For this review, take the finished solid that the model builds, in its own axes (mm). A direction names the side the tool comes from. Coordinates: 2 decimals unless noted, no trailing zeros. Write each loop counter-clockwise with the first axis right and the second up, starting at its lowest first coordinate (ties: lowest second). Pieces come first, ordered by that corner, then holes. Notation, with made-up numbers: (19, 17) -> (32, 17) arc R35 ccw to (32, 55) -> close; hole circle Ø8 at (79.5, 87.25). An arc over 180 degrees is marked (long way). Put each result on its own line as item: value. Start each with the question number.
Item 1: To check wall thickness, follow L1, parallel to Y at x = -43.5, z = -18.5; L2, parallel to Z at x = -38.5, y = 4.25; L3, parallel to X at y = -1.25, z = -8. State the ranges of each line that lie inside material, in increasing order.
Item 2: For faces 4 (the flat face through (-21, 5, -17)), 5 (the flat face through (-37, 2, -24)), 6 (the flat face through (-40.7, 0, -14.2)), list the 3-axis set-ups (+Z, -Z, +X, -X, +Y, -Y) from which the entire face can be reached by the end or side of a thin tool; tool diameter is ignored.
Item 3: Consider section C-C on y = -6.75. Give the boundary of the cut face in (x, z).
Item 4: The part is to be moulded in two halves that separate along X. For faces 1 (the flat face through (0, -2, -17)), 2 (the flat face through (-38, 2, -4)), 3 (the cylindrical face through (-29.141, 2.535, -25.203)), say which applies: +X half, -X half, draft (parallel to the pull), parting line (faces both ways), or undercut.
Item 5: Consider section D-D on z = -30. Give the boundary of the cut face in (x, y).
Item 6: Consider section B-B on z = -18. Give the boundary of the cut face in (x, y), and give its area (3 significant figures).
Item 7: Insertion check: P1, Ø4, axis at x = -38.5, y = 1.5, coming from the +Z side; P2, Ø1.5, axis at y = -4, z = -23, coming from the -X side; P3, Ø2.5, axis at x = -35.5, y = 3, coming from the -Z side. Each pin has a flat end and moves straight along its axis. Give the tip position at first contact, or say it passes through.
```python
from build123d import *

# Parameters (mm, degrees)
AUFSATZ_LINEAR_AUSTRAGEN1_DEPTH = 5
SKIZZE4_W                       = 28
SKIZZE4_H                       = 33
AUFSATZ_LINEAR_AUSTRAGEN3_DEPTH = 10
VERRUNDUNG1_R                   = 4
VERRUNDUNG2_R                   = 4


with BuildPart() as part:
    # Skizze2 → Aufsatz-Linear austragen1 (new body)
    with BuildSketch(Plane(origin=(0, 0, 0), x_dir=(1, 0, 0), z_dir=(0, 1, 0))):
        with BuildLine():
            Line((0, 33), (-28, 33))
            Line((-28, 33), (-28, 24))
            Line((-28, 24), (-43, 24))
            ThreePointArc((-43, 24), (-35.928932188, 21.071067812), (-33, 14))
            ThreePointArc((-33, 14), (-35.928932188, 6.928932188), (-43, 4))
            Line((-43, 4), (-28, 4))
            Line((-28, 4), (-28, 0))
            Line((-28, 0), (0, 0))
            Line((0, 0), (0, 33))
        make_face()
        with BuildLine():
            ThreePointArc((-33, 14), (-35.928932188, 21.071067812), (-43, 24))
            Line((-43, 24), (-43, 16))
            ThreePointArc((-43, 16), (-41.585786438, 15.414213562), (-41, 14))
            ThreePointArc((-41, 14), (-41.585786438, 12.585786438), (-43, 12))
            Line((-43, 12), (-43, 4))
            ThreePointArc((-43, 4), (-35.928932188, 6.928932188), (-33, 14))
        make_face()
        with BuildLine():
            Line((-43, 16), (-43, 24))
            ThreePointArc((-43, 24), (-53, 14), (-43, 4))
            Line((-43, 4), (-43, 12))
            ThreePointArc((-43, 12), (-45, 14), (-43, 16))
        make_face()
    extrude(amount=AUFSATZ_LINEAR_AUSTRAGEN1_DEPTH)

    # Skizze4 → Aufsatz-Linear austragen3 (add)
    with BuildSketch(Plane.XZ):
        with Locations((-14, -16.5)):
            Rectangle(SKIZZE4_W, SKIZZE4_H)
    extrude(amount=AUFSATZ_LINEAR_AUSTRAGEN3_DEPTH)

    # Verrundung1
    verrundung1_edges = [part.edges().sort_by_distance(p)[0] for p in [
        (-28, 2.5, -4),
    ]]
    fillet(verrundung1_edges, radius=VERRUNDUNG1_R - 0.0001)  # a hair under: the kernel refuses the full size

    # Verrundung2
    verrundung2_edges = [part.edges().sort_by_distance(p)[0] for p in [
        (-28, 2.5, -24),
    ]]
    fillet(verrundung2_edges, radius=VERRUNDUNG2_R)


solid = part.part
```
Return value:
1. L1: 0 to 5
1. L2: -24 to -4
1. L3: -28 to 0
2. face 4: +Z, -Z, +X, -X, +Y
2. face 5: -Z, -X, +Y, -Y
2. face 6: +Z, -Z, -X, -Y
3. outline: (-28, -33) -> (0, -33) -> (0, 0) -> (-28, 0) -> close
4. face 1: +X half
4. face 2: draft
4. face 3: -X half
5. outline: (-28, -10) -> (0, -10) -> (0, 5) -> (-28, 5) -> close
6. outline: (-52.17, 0) -> (-28, 0) -> (-28, -10) -> (0, -10) -> (0, 5) -> (-52.17, 5) -> close
6. area: 541 mm^2
7. P1: z = -4
7. P2: x = -28
7. P3: z = -24
